Could you check a few things on this model? Use its own coordinates, in mm. A direction names the side the tool comes from. Round coordinates to 2 decimals unless told otherwise and drop trailing zeros. Write each loop counter-clockwise with the first axis right and the second up, starting at its lowest first coordinate (ties: lowest second). Pieces come first, ordered by that corner, then holes. Notation, with made-up numbers: (24.5, 78.5) -> (72.5, 78.5) arc R6 cw to (72.5, 82.5) -> close; hole circle Ø3 at (14.5, 9). An arc over 180 degrees is marked (long way). Answer in a Markdown table with one row per item.
Autodesk Fusion 360 part; units mm, degrees
sketch "Sketch1" plane through (0, 0, 0) normal (0, 1, 0) x (1, 0, 0)
  line L0 (0, 0) -> (76.2, 0)
  line L1 (76.2, 0) -> (76.2, 25.4)
  line L2 (76.2, 25.4) -> (0, 25.4)
  line L3 (0, 25.4) -> (0, 0)
  dimension "d1" = 76.2
  dimension "d2" = 25.4
extrude "Extrude1" add sketch "Sketch1" along normal blind 25.4
sketch "Sketch2" plane through (0, 25.4, 0) normal (0, 1, 0) x (-1, 0, 0)
  line L0 (0, -25.4) -> (0, 0)
  line L1 (0, 0) -> (-76.2, 0)
  line L2 (-76.2, 0) -> (-76.2, -25.4)
  line L3 (-76.2, -25.4) -> (0, -25.4)
  circle A0 centre (-18.1, -12.7) radius 6.096
  circle A1 centre (-58.1, -12.7) radius 6.096
  dimension "d6" = 12.192
  dimension "d8" = 12.192
extrude "Extrude2" add sketch "Sketch2" along normal blind 4 contours A0 | A1
sketch "Sketch3" plane through (0, 29.4, 0) normal (0, 1, 0) x (-1, 0, 0)
  circle A0 centre (-18.1, -12.7) radius 6.096
  circle A1 centre (-18.1, -12.7) radius 2.3813
  dimension "d11" = 4.7625
extrude "Extrude3" cut sketch "Sketch3" against normal blind 12.7 contours A1
sketch "Sketch4" plane through (0, 29.4, 0) normal (0, 1, 0) x (-1, 0, 0)
  circle A0 centre (-58.1, -12.7) radius 6.096
  circle A1 centre (-58.1, -12.7) radius 2.3813
  dimension "d14" = 4.7625
extrude "Extrude4" cut sketch "Sketch4" against normal blind 12.7 contours A1
1) For pin 1 (1.4 mm diameter, centred on x = 57.5, z = -12, fed in from +Y), with a flat end and sliding along its axis, tell me the tip position at first contact or that it passes through.
Findings:
| item | result |
|---|---|
| pin 1 | stops at y = 16.7 |
2) Please list where these lines run through material, in increasing order: line 1 (Z direction, x = 58.1, y = 20.75); line 2 (X direction, y = 24.75, z = -14.5); line 3 (Z direction, x = 18.1, y = 25.75).
Findings:
| item | result |
|---|---|
| line 1 | z = -25.4 to -15.08, -10.32 to 0 |
| line 2 | x = 0 to 16.54, 19.66 to 56.54, 59.66 to 76.2 |
| line 3 | z = -18.8 to -15.08, -10.32 to -6.6 |
3) For faces 1 (the face through (76.2, 13, -13)), 2 (the face through (60.48, 23.14, -12.6)), which set-ups out of +Z, -Z, +X, -X, +Y, -Y let a thin tool reach every point of the face, with its end or its side?
Findings:
| item | result |
|---|---|
| face 1 | +Z, -Z, +X, +Y, -Y |
| face 2 | +Y |
4) Imagine slicing it at B-B, the plane z = -12.7. Please give me the cut outline in (x, y), plus the area to 3 significant figures.
Findings:
| item | result |
|---|---|
| outline | (0, 0) -> (76.2, 0) -> (76.2, 25.4) -> (64.2, 25.4) -> (64.2, 29.4) -> (60.48, 29.4) -> (60.48, 16.7) -> (55.72, 16.7) -> (55.72, 29.4) -> (52, 29.4) -> (52, 25.4) -> (24.2, 25.4) -> (24.2, 29.4) -> (20.48, 29.4) -> (20.48, 16.7) -> (15.72, 16.7) -> (15.72, 29.4) -> (12, 29.4) -> (12, 25.4) -> (0, 25.4) -> close |
| area | 1,910 mm^2 |
5) Imagine slicing it at C-C, the plane x = 54.5. Please give me the cut outline in (y, z).
Findings:
| item | result |
|---|---|
| outline | (0, -25.4) -> (25.4, -25.4) -> (25.4, -17.62) -> (29.4, -17.62) -> (29.4, -7.78) -> (25.4, -7.78) -> (25.4, 0) -> (0, 0) -> close |
6) Imagine slicing it at A-A, the plane x = 18.1. Please give me the cut outline in (y, z).
Findings:
| item | result |
|---|---|
| outline | (0, -25.4) -> (25.4, -25.4) -> (25.4, -18.8) -> (29.4, -18.8) -> (29.4, -15.08) -> (16.7, -15.08) -> (16.7, -10.32) -> (29.4, -10.32) -> (29.4, -6.6) -> (25.4, -6.6) -> (25.4, 0) -> (0, 0) -> close |
7) Imagine slicing it at D-D, the plane z = -9.5. Please give me the cut outline in (x, y), plus the area to 3 significant figures.
Findings:
| item | result |
|---|---|
| outline | (0, 0) -> (76.2, 0) -> (76.2, 25.4) -> (63.29, 25.4) -> (63.29, 29.4) -> (52.91, 29.4) -> (52.91, 25.4) -> (23.29, 25.4) -> (23.29, 29.4) -> (12.91, 29.4) -> (12.91, 25.4) -> (0, 25.4) -> close |
| area | 2,020 mm^2 |
8) Thinking about a two-plate mould opening in Z: for faces 3 (the face through (15.83, 23.14, -11.98)), 4 (the face through (15, 29.4, -13)), 5 (the face through (52.286, 27.372, -14.531)), which applies, +Z half, -Z half, draft (parallel to the pull), parting line (faces both ways), or undercut?
Findings:
| item | result |
|---|---|
| face 3 | undercut |
| face 4 | draft |
| face 5 | parting line |
